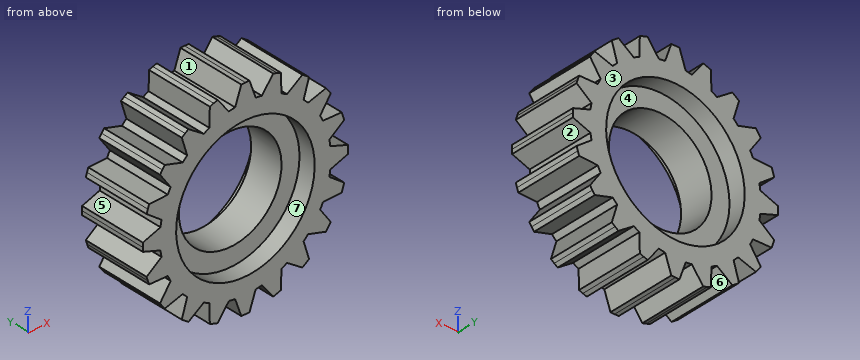
from build123d import *

# Parameters (mm, degrees)
SKETCH1_R           = 20.25
BOSS_EXTRUDE1_DEPTH = 10
SKETCH1_3_R         = 20.25
SKETCH1_3_R_2       = 15
BOSS_EXTRUDE2_DEPTH = 5


with BuildPart() as part:
    # Sketch1 → Boss-Extrude1 (new, symmetric)
    with BuildSketch(Plane(origin=(0, 0, 0), x_dir=(1, 0, 0), z_dir=(0, 1, 0))):
        with BuildLine():
            Line((30, 0), (29.976, 1.199759976))
            Line((29.976, 1.199759976), (24.819347292, 3))
            ThreePointArc((24.819347292, 3), (24.692208515, 3.910861626), (24.531652955, 4.816430554))
            Line((24.531652955, 4.816430554), (28.879616354, 8.12205388))
            Line((28.879616354, 8.12205388), (28.531695489, 9.270509831))
            Line((28.531695489, 9.270509831), (28.138123911, 10.404132967))
            Line((28.138123911, 10.404132967), (22.677550989, 10.522769651))
            ThreePointArc((22.677550989, 10.522769651), (22.275163105, 11.349762493), (21.842629505, 12.161395327))
            Line((21.842629505, 12.161395327), (24.956294644, 16.648824513))
            Line((24.956294644, 16.648824513), (24.270509831, 17.633557569))
            Line((24.270509831, 17.633557569), (23.545892203, 18.590076932))
            Line((23.545892203, 18.590076932), (18.315917992, 17.015497293))
            ThreePointArc((18.315917992, 17.015497293), (17.67766953, 17.67766953), (17.015497293, 18.315917992))
            Line((17.015497293, 18.315917992), (18.590076932, 23.545892203))
            Line((18.590076932, 23.545892203), (17.633557569, 24.270509831))
            Line((17.633557569, 24.270509831), (16.648824513, 24.956294644))
            Line((16.648824513, 24.956294644), (12.161395327, 21.842629505))
            ThreePointArc((12.161395327, 21.842629505), (11.349762493, 22.275163105), (10.522769651, 22.677550989))
            Line((10.522769651, 22.677550989), (10.404132967, 28.138123911))
            Line((10.404132967, 28.138123911), (9.270509831, 28.531695489))
            Line((9.270509831, 28.531695489), (8.12205388, 28.879616354))
            Line((8.12205388, 28.879616354), (4.816430554, 24.531652955))
            ThreePointArc((4.816430554, 24.531652955), (3.910861626, 24.692208515), (3, 24.819347292))
            Line((3, 24.819347292), (1.199759976, 29.976))
            Line((1.199759976, 29.976), (0, 30))
            Line((0, 30), (-1.199759976, 29.976))
            Line((-1.199759976, 29.976), (-3, 24.819347292))
            ThreePointArc((-3, 24.819347292), (-3.910861626, 24.692208515), (-4.816430554, 24.531652955))
            Line((-4.816430554, 24.531652955), (-8.12205388, 28.879616354))
            Line((-8.12205388, 28.879616354), (-9.270509831, 28.531695489))
            Line((-9.270509831, 28.531695489), (-10.404132967, 28.138123911))
            Line((-10.404132967, 28.138123911), (-10.522769651, 22.677550989))
            ThreePointArc((-10.522769651, 22.677550989), (-11.349762493, 22.275163105), (-12.161395327, 21.842629505))
            Line((-12.161395327, 21.842629505), (-16.648824513, 24.956294644))
            Line((-16.648824513, 24.956294644), (-17.633557569, 24.270509831))
            Line((-17.633557569, 24.270509831), (-18.590076932, 23.545892203))
            Line((-18.590076932, 23.545892203), (-17.015497293, 18.315917992))
            ThreePointArc((-17.015497293, 18.315917992), (-17.67766953, 17.67766953), (-18.315917992, 17.015497293))
            Line((-18.315917992, 17.015497293), (-23.545892203, 18.590076932))
            Line((-23.545892203, 18.590076932), (-24.270509831, 17.633557569))
            Line((-24.270509831, 17.633557569), (-24.956294644, 16.648824513))
            Line((-24.956294644, 16.648824513), (-21.842629505, 12.161395327))
            ThreePointArc((-21.842629505, 12.161395327), (-22.275163105, 11.349762493), (-22.677550989, 10.522769651))
            Line((-22.677550989, 10.522769651), (-28.138123911, 10.404132967))
            Line((-28.138123911, 10.404132967), (-28.531695489, 9.270509831))
            Line((-28.531695489, 9.270509831), (-28.879616354, 8.12205388))
            Line((-28.879616354, 8.12205388), (-24.531652955, 4.816430554))
            ThreePointArc((-24.531652955, 4.816430554), (-24.692208515, 3.910861626), (-24.819347292, 3))
            Line((-24.819347292, 3), (-29.976, 1.199759976))
            Line((-29.976, 1.199759976), (-30, 0))
            Line((-30, 0), (-29.976, -1.199759976))
            Line((-29.976, -1.199759976), (-24.819347292, -3))
            ThreePointArc((-24.819347292, -3), (-24.692208515, -3.910861626), (-24.531652955, -4.816430554))
            Line((-24.531652955, -4.816430554), (-28.879616354, -8.12205388))
            Line((-28.879616354, -8.12205388), (-28.531695489, -9.270509831))
            Line((-28.531695489, -9.270509831), (-28.138123911, -10.404132967))
            Line((-28.138123911, -10.404132967), (-22.677550989, -10.522769651))
            ThreePointArc((-22.677550989, -10.522769651), (-22.275163105, -11.349762493), (-21.842629505, -12.161395327))
            Line((-21.842629505, -12.161395327), (-24.956294644, -16.648824513))
            Line((-24.956294644, -16.648824513), (-24.270509831, -17.633557569))
            Line((-24.270509831, -17.633557569), (-23.545892203, -18.590076932))
            Line((-23.545892203, -18.590076932), (-18.315917992, -17.015497293))
            ThreePointArc((-18.315917992, -17.015497293), (-17.67766953, -17.67766953), (-17.015497293, -18.315917992))
            Line((-17.015497293, -18.315917992), (-18.590076932, -23.545892203))
            Line((-18.590076932, -23.545892203), (-17.633557569, -24.270509831))
            Line((-17.633557569, -24.270509831), (-16.648824513, -24.956294644))
            Line((-16.648824513, -24.956294644), (-12.161395327, -21.842629505))
            ThreePointArc((-12.161395327, -21.842629505), (-11.349762493, -22.275163105), (-10.522769651, -22.677550989))
            Line((-10.522769651, -22.677550989), (-10.404132967, -28.138123911))
            Line((-10.404132967, -28.138123911), (-9.270509831, -28.531695489))
            Line((-9.270509831, -28.531695489), (-8.12205388, -28.879616354))
            Line((-8.12205388, -28.879616354), (-4.816430554, -24.531652955))
            ThreePointArc((-4.816430554, -24.531652955), (-3.910861626, -24.692208515), (-3, -24.819347292))
            Line((-3, -24.819347292), (-1.199759976, -29.976))
            Line((-1.199759976, -29.976), (0, -30))
            Line((0, -30), (1.199759976, -29.976))
            Line((1.199759976, -29.976), (3, -24.819347292))
            ThreePointArc((3, -24.819347292), (3.910861626, -24.692208515), (4.816430554, -24.531652955))
            Line((4.816430554, -24.531652955), (8.12205388, -28.879616354))
            Line((8.12205388, -28.879616354), (9.270509831, -28.531695489))
            Line((9.270509831, -28.531695489), (10.404132967, -28.138123911))
            Line((10.404132967, -28.138123911), (10.522769651, -22.677550989))
            ThreePointArc((10.522769651, -22.677550989), (11.349762493, -22.275163105), (12.161395327, -21.842629505))
            Line((12.161395327, -21.842629505), (16.648824513, -24.956294644))
            Line((16.648824513, -24.956294644), (17.633557569, -24.270509831))
            Line((17.633557569, -24.270509831), (18.590076932, -23.545892203))
            Line((18.590076932, -23.545892203), (17.015497293, -18.315917992))
            ThreePointArc((17.015497293, -18.315917992), (17.67766953, -17.67766953), (18.315917992, -17.015497293))
            Line((18.315917992, -17.015497293), (23.545892203, -18.590076932))
            Line((23.545892203, -18.590076932), (24.270509831, -17.633557569))
            Line((24.270509831, -17.633557569), (24.956294644, -16.648824513))
            Line((24.956294644, -16.648824513), (21.842629505, -12.161395327))
            ThreePointArc((21.842629505, -12.161395327), (22.275163105, -11.349762493), (22.677550989, -10.522769651))
            Line((22.677550989, -10.522769651), (28.138123911, -10.404132967))
            Line((28.138123911, -10.404132967), (28.531695489, -9.270509831))
            Line((28.531695489, -9.270509831), (28.879616354, -8.12205388))
            Line((28.879616354, -8.12205388), (24.531652955, -4.816430554))
            ThreePointArc((24.531652955, -4.816430554), (24.692208515, -3.910861626), (24.819347292, -3))
            Line((24.819347292, -3), (29.976, -1.199759976))
            Line((29.976, -1.199759976), (30, 0))
        make_face()
        with Locations(Location((0, 0, 0), (0, 0, 270))):
            Circle(SKETCH1_R, mode=Mode.SUBTRACT)
    extrude(amount=BOSS_EXTRUDE1_DEPTH, both=True)

    # Sketch1_3 → Boss-Extrude2 (add, symmetric)
    with BuildSketch(Plane(origin=(0, 0, 0), x_dir=(1, 0, 0), z_dir=(0, 1, 0))):
        with Locations(Location((0, 0, 0), (0, 0, 270))):
            Circle(SKETCH1_3_R)
        with Locations(Location((0, 0, 0), (0, 0, 270))):
            Circle(SKETCH1_3_R_2, mode=Mode.SUBTRACT)
    extrude(amount=BOSS_EXTRUDE2_DEPTH, both=True)


solid = part.part
Here's how the part is built. I have some questions about the finished solid (model axes, mm). Face numbers are marked on the shaded views. A direction names the side the tool comes from. Round coordinates to 2 decimals unless told otherwise and drop trailing zeros. Order: outer loops, then holes, each group sorted by start corner. A loop starts at its lowest first (then second) coordinate and runs counter-clockwise, first axis right, second up. Notation, with made-up numbers: M 28.5,63 L 84.5,63 A12 ccw 84.5,73 Z; hole C -28,87 d5. An arc over 180 degrees is marked long. One line per question, with ' | ' between items.
1) On a 3-axis mill with a long thin cutter (end or side, diameter ignored), from which of +Z, -Z, +X, -X, +Y, -Y can I reach the whole of each face in a straight line? I mean the marked faces 5, 6 and 7. Say none if no direction works.
Checked values:
face 5: -X, +Y, -Y | face 6: -Z, +Y, -Y | face 7: -Y
2) I need wall thicknesses on line 1 (Z direction, x = 23.5, y = -3.75); line 2 (X direction, y = -2.75, z = 22.5); line 3 (X direction, y = -8.7, z = 0). Which ranges of each line are inside material? Lowest first, please.
Checked values:
line 1: z = -18.58 to -14.55, -10.5 to 10.5, 14.55 to 18.58 | line 2: x = -18.28 to -13.11, -10.9 to 10.9, 13.11 to 18.28 | line 3: x = -30 to -20.25, 20.25 to 30
3) I'm going to push flat-ended pins straight in: pin 1 Ø6 at (y, z) = (7.5, -3.5) entering from +X; pin 2 Ø1 at (x, y) = (-14.5, 2) entering from +Z; pin 3 Ø2 at (x, y) = (-7, -2.5) entering from -Z; pin 4 Ø24 at (x, z) = (0, 0) entering from -Y. Where does each tip first touch, or does it pass through?
Checked values:
pin 1: stops at x = 29.99 | pin 2: stops at z = 23.81 | pin 3: stops at z = -28.72 | pin 4: passes through
4) We'd pull the mould along X, two halves only. Please class the marked faces 1, 2, 3 and 4: released by +X, released by -X, zero draft, split by the parting line, or undercut.
Checked values:
face 1: undercut | face 2: released by +X | face 3: zero draft | face 4: undercut
5) Imagine slicing it at A-A, the plane z = 26. Write out the boundary of the cut face in (x, y).
Checked values:
outline: M -10.45,-10 L -5.93,-10 L -5.93,10 L -10.45,10 Z; M -2.59,-10 L 2.59,-10 L 2.59,10 L -2.59,10 Z; M 5.93,-10 L 10.45,-10 L 10.45,10 L 5.93,10 Z
